```python
from build123d import *

# Parameters (mm, degrees)
SKETCH2_R                 = 1.1303
BOSS_EXTRUDE3_DEPTH       = 1.5875
SKETCH4_R                 = 1.9986
SKETCH4_R_2               = 2.3
CUT_EXTRUDE1_DEPTH        = 55.106562968
SKETCH3_W                 = 58.8
SKETCH3_H                 = 35.28
CUT_EXTRUDE2_DEPTH        = 55.106562968
TAP_DRILL_FOR_4_40_TAP1_D = 2.2606


with BuildPart() as part:
    # Sketch2 → Boss-Extrude3 (new body)
    with BuildSketch(Plane(origin=(0, 0, 0), x_dir=(1, 0, 0), z_dir=(0, 1, 0))):
        with BuildLine():
            Line((-45, 25.825), (-45, -25.825))
            ThreePointArc((-45, -25.825), (-43.777170811, -28.777170811), (-40.825, -30))
            Line((-40.825, -30), (40.825, -30))
            ThreePointArc((40.825, -30), (43.777170811, -28.777170811), (45, -25.825))
            Line((45, -25.825), (45, 25.825))
            ThreePointArc((45, 25.825), (43.777170811, 28.777170811), (40.825, 30))
            Line((40.825, 30), (-40.825, 30))
            ThreePointArc((-40.825, 30), (-43.777170811, 28.777170811), (-45, 25.825))
        make_face()
        with Locations(Location((40.825, 25.825, 0), (0, 0, 270))):
            Circle(SKETCH2_R, mode=Mode.SUBTRACT)
        with Locations(Location((40.825, -25.825, 0), (0, 0, 270))):
            Circle(SKETCH2_R, mode=Mode.SUBTRACT)
        with Locations(Location((-40.825, 25.825, 0), (0, 0, 270))):
            Circle(SKETCH2_R, mode=Mode.SUBTRACT)
        with Locations(Location((-40.825, -25.825, 0), (0, 0, 270))):
            Circle(SKETCH2_R, mode=Mode.SUBTRACT)
    extrude(amount=BOSS_EXTRUDE3_DEPTH)

    # Sketch4 → Cut-Extrude1 (cut, through all)
    with BuildSketch(Plane(origin=(0, 1.5875, 0), x_dir=(1, 0, 0), z_dir=(0, 1, 0))):
        with Locations(Location((-33.825, 14.109, 0), (0, 0, 270))):
            Circle(SKETCH4_R)
        with Locations(Location((-33.825, 7.053, 0), (0, 0, 270))):
            Circle(SKETCH4_R_2)
        with Locations(Location((-33.825, -0.003, 0), (0, 0, 270))):
            Circle(SKETCH4_R_2)
        with Locations(Location((-33.825, -7.059, 0), (0, 0, 270))):
            Circle(SKETCH4_R_2)
        with Locations(Location((-33.825, -14.115, 0), (0, 0, 270))):
            Circle(SKETCH4_R_2)
    extrude(amount=-CUT_EXTRUDE1_DEPTH, mode=Mode.SUBTRACT)

    # Sketch3 → Cut-Extrude2 (cut, through all)
    with BuildSketch(Plane(origin=(0, 1.5875, 0), x_dir=(1, 0, 0), z_dir=(0, 1, 0))):
        with Locations((3.24, 0)):
            Rectangle(SKETCH3_W, SKETCH3_H)
    extrude(amount=-CUT_EXTRUDE2_DEPTH, mode=Mode.SUBTRACT)

    # Tap Drill for #4-40 Tap1 (through all)
    with Locations(Plane(origin=(-40.825, 1.5875, 25.825), x_dir=(0, 0, 1), z_dir=(0, 1, 0))):
        with Locations((0, 0), (-51.65, 0), (-51.65, 81.65), (0, 81.65)):
            Hole(TAP_DRILL_FOR_4_40_TAP1_D / 2)


solid = part.part
```
Design review of the part built by this model. Coordinates are the model's own, in mm. Coordinates: 2 decimals unless noted, no trailing zeros. Order: outer loops, then holes, each group sorted by start corner. A loop starts at its lowest first (then second) coordinate and runs counter-clockwise, first axis right, second up.
1) Take a section at A-A, the plane z = 3.5. Give the boundary of the cut face in (x, y), and give its area (3 significant figures).
2) Take a section at D-D, the plane y = 1.2. State how many separate pieces and enclosed holes the cut face has, and give its area (3 significant figures).
3) Take a section at B-B, the plane x = -2. Give the boundary of the cut face in (y, z).
4) Mouldability with a two-part tool opening along X and no side actions: class faces 1 (the cylindrical face through (-41.93, 0.78, -26.07)), 2 (the flat face through (-1, 1.588, -20)), 3 (the cylindrical face through (-43.745, 0.783, -28.809)) as +X half, -X half, draft (parallel to the pull), parting line (faces both ways), or undercut.
5) Wall thickness on line 1 along X through (y, z) = (1.55, -26); line 2 along X through (y, z) = (0.3, 0) (3 decimals); line 3 along Z through (x, y) = (41, 1.4): over which ranges is each line inside the solid? List them lowest first.
6) Take a section at C-C, the plane z = 13. Give the boundary of the cut face in (x, y), and give its area (3 significant figures).
Returned:
1. outline: (-45, 0) - (-26.16, 0) - (-26.16, 1.59) - (-45, 1.59) - close; (32.64, 0) - (45, 0) - (45, 1.59) - (32.64, 1.59) - close
1. area: 49.5 mm2
2. separate pieces: 1
2. enclosed holes: 10
2. area: 3,220 mm2
3. outline: (0, -30) - (1.59, -30) - (1.59, -17.64) - (0, -17.64) - close; (0, 17.64) - (1.59, 17.64) - (1.59, 30) - (0, 30) - close
4. face 1: undercut
4. face 2: draft
4. face 3: -X half
5. line 1: x = -45 to -41.94, -39.71 to 39.71, 41.94 to 45
5. line 2: x = -45 to -36.125, -31.525 to -26.16, 32.64 to 45
5. line 3: z = -30 to -26.94, -24.71 to 24.71, 26.94 to 30
6. outline: (-45, 0) - (-35.84, 0) - (-35.84, 1.59) - (-45, 1.59) - close; (-31.81, 0) - (-26.16, 0) - (-26.16, 1.59) - (-31.81, 1.59) - close; (32.64, 0) - (45, 0) - (45, 1.59) - (32.64, 1.59) - close
6. area: 43.1 mm2
